Can you work these out from the model? Positions are in its coordinate system, mm. A direction names the side the tool comes from. Coordinates: 2 decimals unless noted, no trailing zeros. Loops run counter-clockwise (first coordinate to the right, second up) from the corner with the lowest first, then second, coordinate; pieces in that order, holes last. Notation, with made-up numbers: M 59,5 L 70,5 A23 ccw 70,32 Z; hole C 42.5,-13.75 d4. An arc over 180 degrees is marked long. Answer as a JSON object with one key per item and string values. Group by question number.
Item 1: If I drill on line 1 (Y direction, x = 0, z = -27); line 2 (Y direction, x = 6.75, z = 8); line 3 (Z direction, x = 0, y = 18.7), over which ranges is the centre line in solid material (lowest first)?
Item 2: Suppose I cut it at B-B (x = 0). Write out the boundary of the cut face in (y, z).
Item 3: Suppose I cut it at C-C (x = 6.5). Count the separate pieces of the cut face and the enclosed holes in it, then the cut area to 3 significant figures.
Item 4: I'm going to push flat-ended pins straight in: pin 1 Ø13 at (x, z) = (0, 0) entering from +Y; pin 2 Ø6 at (x, y) = (1.5, 9) entering from -Z; pin 3 Ø1.5 at (x, y) = (5.5, 10.5) entering from +Z; pin 4 Ø2 at (x, y) = (-3, 3) entering from +Z. Where does each tip first touch, or does it pass through?
Item 5: We'd pull the mould along X, two halves only. Please class faces 3 (the flat face through (-10.986, 11, -21)), 4 (the cylindrical face through (-7.067, 19.848, -1.569)), 5 (the flat face through (0, 22.276, -14)): +X half, -X half, draft (parallel to the pull), parting line (faces both ways), or undercut.
Item 6: Which directions (+Z, -Z, +X, -X, +Y, -Y) give clear straight access to the entire face, cutting with the end or side of a thin tool? Please do faces 1 (the cylindrical face through (0.242, 2.36, 10.983)), 2 (the flat face through (0, 17.488, -8)).
Item 7: Suppose I cut it at A-A (z = -19.5). Write out the boundary of the cut face in (x, y), then the cut area to 3 significant figures.
```python
from build123d import *

# Parameters (mm, degrees)
SKETCH1_R           = 7.239
BOSS_EXTRUDE1_DEPTH = 22.2758
SKETCH2_W           = 31.5468
SKETCH2_H           = 12.7
CUT_EXTRUDE1_DEPTH  = 12.7
CUT_EXTRUDE2_REACH  = 52.741
SKETCH7_R           = 3.81


with BuildPart() as part:
    # Sketch1 → Boss-Extrude1 (new body)
    with BuildSketch(Plane(origin=(0, 0, 0), x_dir=(1, 0, 0), z_dir=(0, 1, 0))):
        with BuildLine():
            Line((-10.9855, 0), (-10.9855, 33.2613))
            Line((-10.9855, 33.2613), (10.9855, 33.2613))
            Line((10.9855, 33.2613), (10.9855, 0))
            ThreePointArc((10.9855, 0), (0, -10.9855), (-10.9855, 0))
        make_face()
        with Locations(Location((0, 0, 0), (0, 0, 270))):
            Circle(SKETCH1_R, mode=Mode.SUBTRACT)
    extrude(amount=BOSS_EXTRUDE1_DEPTH)

    # Sketch2 → Cut-Extrude1 (cut, symmetric)
    with BuildSketch(Plane(origin=(0, 0, 0), x_dir=(0, 0, -1), z_dir=(1, 0, 0))):
        with Locations((4.7879, 11.1379)):
            Rectangle(SKETCH2_W, SKETCH2_H)
    extrude(amount=CUT_EXTRUDE1_DEPTH, both=True, mode=Mode.SUBTRACT)

    # Sketch5 → Cut-Revolve1 (revolve, cut)
    with BuildSketch(Plane(origin=(5.568421495, 5.492228727, 0), x_dir=(0, 0, 1), z_dir=(-0.7119608885898049, -0.7022191204449046, 0)), mode=Mode.PRIVATE) as cut_revolve1_sk:
        Polygon((-21.436464447, 23.57372651), (-33.2613, 16.184749181), (-33.2613, 23.57372651), align=None)
    revolve(cut_revolve1_sk.sketch.rotate(Axis((0, 11.1379, -33.2613), (0, 0, 1)), 270.789356568), axis=Axis((0, 11.1379, -33.2613), (0, 0, 1)), mode=Mode.SUBTRACT)

    # Sketch7 → Cut-Extrude2 (cut, up to next)
    with BuildSketch(Plane(origin=(0, 0, -33.2613), x_dir=(-1, 0, 0), z_dir=(0, 0, -1)), mode=Mode.PRIVATE) as cut_extrude2_sk1:
        with Locations((0, 11.1379)):
            Circle(SKETCH7_R)
    cut_extrude2_tool1 = extrude(cut_extrude2_sk1.sketch, amount=-CUT_EXTRUDE2_REACH, mode=Mode.PRIVATE) & part.part
    add(cut_extrude2_tool1.solids().sort_by_distance((0, 11.1379, -33.2613))[0], mode=Mode.SUBTRACT)


solid = part.part
```
From the geometry:
{
 "1": {"line 1": "0 to 7.33, 14.95 to 22.28", "line 2": "0 to 4.79, 17.49 to 22.28", "line 3": "-33.26 to -7.24, 7.24 to 10.99"},
 "2": {"outline": "M 0,-28.65 L 2.88,-33.26 L 7.33,-33.26 L 7.33,-20.56 L 4.79,-20.56 L 4.79,-7.24 L 0,-7.24 Z; M 0,7.24 L 4.79,7.24 L 4.79,10.99 L 0,10.99 Z; M 14.95,-33.26 L 19.39,-33.26 L 22.28,-28.65 L 22.28,-7.24 L 17.49,-7.24 L 17.49,-20.56 L 14.95,-20.56 Z; M 17.49,7.24 L 22.28,7.24 L 22.28,10.99 L 17.49,10.99 Z"},
 "3": {"separate pieces": "3", "enclosed holes": "0", "area": "461 mm2"},
 "4": {"pin 1": "through", "pin 2": "z = -33.26", "pin 3": "z = -20.56", "pin 4": "z = 10.8"},
 "5": {"face 3": "-X half", "face 4": "undercut", "face 5": "draft"},
 "6": {"face 1": "+Z, +Y, -Y", "face 2": "+Z, +X, -X"},
 "7": {"outline": "M -10.99,0 L 10.99,0 L 10.99,4.79 L -10.99,4.79 Z; M -10.99,17.49 L 10.99,17.49 L 10.99,22.28 L -10.99,22.28 Z", "area": "210 mm2"}
}
